Read the model definition and answer for the solid it produces. Units are mm, in the model's axes. A direction names the side the tool comes from. Coordinates: 2 decimals unless noted, no trailing zeros. Loops run counter-clockwise (first coordinate to the right, second up) from the corner with the lowest first, then second, coordinate; pieces in that order, holes last. Notation, with made-up numbers: (0, 15.5) -> (54, 15.5) arc R10 cw to (54, 32.5) -> close; hole circle Ø8 at (21, 6). An arc over 180 degrees is marked (long way). Answer in a Markdown table with one row per item.
```python
from build123d import *

# Parameters (mm, degrees)
F1_DEPTH    = 25
F2_T1_DEPTH = 46.6847527524
F3_SIZE     = 12.99999


# Not quite as in the source:
# - a fillet or chamfer that OpenCascade refuses, or shapes differently, is made with other operations: its cross-section is extruded or revolved along the edge and cut away or added
# - a fillet or chamfer is up to 0.001 mm smaller than in the source, because OpenCascade refuses the exact size


with BuildPart() as f1:
    # F0 (on Front) → F1 (new body)
    with BuildSketch(Plane.XZ):
        Polygon((21.2132034356, 21.2132034356), (0, 0), (134.3502884254, 0), (84.8528137424, 49.4974746831), (75.660425587, 40.3050865276), (66.4680374315, 31.1126983722), (56.5685424949, 21.2132034356), (38.8908729653, 3.5355339059), align=None)
        Polygon((66.4680374315, 31.1126983722), (75.660425587, 40.3050865276), (66.4680374315, 49.4974746831), (57.2756492761, 40.3050865276), align=None)
    extrude(amount=F1_DEPTH)

    # F2: chamfer of 6 x 13 on 2 edges, made by hand

    # F2_s2 → F2_t1 (cut)
    with BuildSketch(Plane(origin=(17.6776695297, 0, -17.6776695297), x_dir=(0, 1, 0), z_dir=(-0.7071067812, 0, 0.7071067812))):
        Polygon((-19, -82), (-25, -69), (-25, -82), align=None)
        Polygon((-6, -82), (0, -69), (0, -82), align=None)
    extrude(amount=F2_T1_DEPTH, mode=Mode.SUBTRACT)

    # F3 (size 13 in the source; OpenCascade refuses exactly that, so slightly less here)
    f3_edges = [f1.edges().sort_by_distance(p)[0] for p in [
        (57.275649, -12.5, 40.305087),
    ]]
    chamfer(f3_edges, length=F3_SIZE)


solid = f1.part
```
1. Find the intervals of material crossed by probe 1 along X at (y, z) = (-4, 16); probe 2 along X at (y, z) = (-15.25, 5.5); probe 3 along Z at (x, y) = (61.5, -1.25), in increasing order.
A:
| item | result |
|---|---|
| probe 1 | x = 16 to 26.43, 51.36 to 118.35 |
| probe 2 | x = 5.5 to 36.93, 40.86 to 128.85 |
| probe 3 | z = 0 to 26.14 |
2. A cutting plane is placed at C-C on x = 20. Give the vertices of the cut face in (y, z), and give its area (3 significant figures).
A:
| item | result |
|---|---|
| outline | (-25, 0) -> (0, 0) -> (0, 20) -> (-25, 20) -> close |
| area | 500 mm2 |
3. Given pin 1 Ø1 at (y, z) = (-8, 38) entering from -X; pin 2 Ø8 at (x, y) = (27.5, -11) entering from +Z; pin 3 Ø1 at (x, y) = (17, -21) entering from +Z, each flat-ended and moving along its own axis, determine where each tip first touches the part or whether it passes through.
A:
| item | result |
|---|---|
| pin 1 | stops at x = 66.47 |
| pin 2 | stops at z = 18.93 |
| pin 3 | stops at z = 17.5 |
4. The mould has two halves that part along X. Classify faces 1 (the flat face through (66.468, -12, 38)), 2 (the flat face through (71.129, -12.409, 44.837)), 3 (the flat face through (66, -25, 14)), 4 (the flat face through (30.176, -12.325, 12.251)): pulls with the +X half, pulls with the -X half, needs draft (parallel to the pull), parting line crosses it, or undercut.
A:
| item | result |
|---|---|
| face 1 | pulls with the -X half |
| face 2 | undercut |
| face 3 | needs draft |
| face 4 | undercut |
5. A cutting plane is placed at D-D on z = 34. Give the vertices of the cut face in (x, y), and give its area (3 significant figures).
A:
| item | result |
|---|---|
| outline | (66.47, -24.06) -> (69.36, -23.12) -> (69.36, -25) -> (100.35, -25) -> (100.35, 0) -> (69.36, 0) -> (69.36, -1.88) -> (66.47, -0.94) -> close |
| area | 839 mm2 |
6. A tool of negligible diameter and unlimited length cuts with its end or side. For faces 5 (the flat face through (68.64, -3.71, 40.31)), 6 (the flat face through (68.64, -21.29, 40.31)), 7 (the flat face through (109.95, -12.32, 24.4)), from which of +Z, -Z, +X, -X, +Y, -Y can it reach the whole face along a straight path? Write none if from no direction.
A:
| item | result |
|---|---|
| face 5 | +Z, +Y |
| face 6 | +Z, -Y |
| face 7 | +Z, +X, +Y, -Y |
7. A cutting plane is placed at B-B on z = 20. Give the vertices of the cut face in (x, y), and give its area (3 significant figures).
A:
| item | result |
|---|---|
| outline | (20, -25) -> (22.43, -25) -> (22.43, 0) -> (20, 0) -> close; (55.36, -25) -> (114.35, -25) -> (114.35, 0) -> (55.36, 0) -> close |
| area | 1,540 mm2 |
